Here's how the part is built. I have some questions about the finished solid (model axes, mm). Face numbers are marked on the shaded views. Round coordinates to 2 decimals unless told otherwise and drop trailing zeros. Loops run counter-clockwise (first coordinate to the right, second up) from the corner with the lowest first, then second, coordinate; pieces in that order, holes last. Notation, with made-up numbers: (60, -19) -> (107, -19) arc R13 ccw to (107, -5) -> close; hole circle Ø1 at (-15, 0). An arc over 180 degrees is marked (long way). Use CSV: the item, a comma, the result in double quotes. Start each with the question number.
from build123d import *

# Parameters (mm, degrees)
SKETCH3_R          = 2
CUT_EXTRUDE1_DEPTH = 5


with BuildPart() as part:
    # Sketch1 → Revolve1 (revolve)
    with BuildSketch(Plane.XY):
        Polygon((-26.75, 0), (-26.400045346, 4), (-20, 4), (-20, 0), align=None)
    revolve(axis=Axis((0, 0, 0), (0, 1, 0)))

    # Sketch3 → Cut-Extrude1 (cut, through all)
    with BuildSketch(Plane.XZ):
        with Locations((-16.263455967, 16.263455967)):
            Circle(SKETCH3_R)
        with Locations((16.263455967, 16.263455967)):
            Circle(SKETCH3_R)
        with Locations((-16.263455967, -16.263455967)):
            Circle(SKETCH3_R)
        with Locations((16.263455967, -16.263455967)):
            Circle(SKETCH3_R)
    extrude(amount=-CUT_EXTRUDE1_DEPTH, mode=Mode.SUBTRACT)


solid = part.part
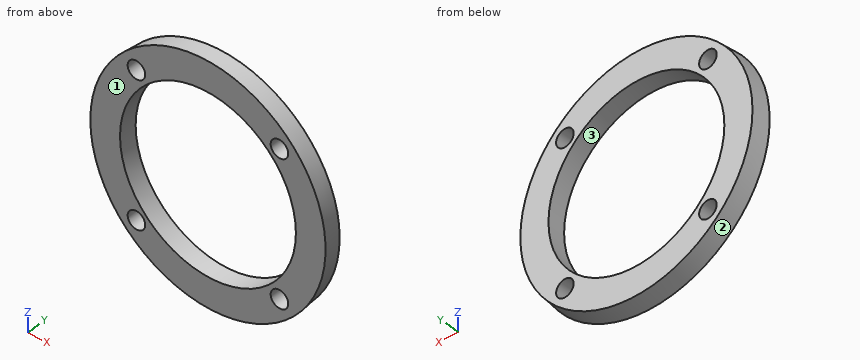
Q1. I need wall thicknesses on line 1 along Z through (x, y) = (-16.5, 0.65); line 2 along X through (y, z) = (0.2, 13.5); line 3 along Z through (x, y) = (9, 3.6). Which ranges of each line are inside material? Lowest first, please.
Q2. I want a section at A-A, the plane x = 0. List the corners of the cut face in (y, z) for me, then the cut area to 3 significant figures.
Q3. I want a section at B-B, the plane z = 0. List the corners of the cut face in (x, y) for me.
Q4. If we mould it in two halves opening along X, with no side actions, what happens to the marked faces 1, 2 and 3? For each: pulls with the +X half, pulls with the -X half, needs draft (parallel to the pull), parting line crosses it, or undercut.
Q5. Will these pins go through, and if not, where does the flat tip stop? pin 1 Ø5 at (x, z) = (15.5, -6.5) entering from +Y; pin 2 Ø2 at (x, y) = (-18.5, 3) entering from -Z; pin 3 Ø1.5 at (x, y) = (12, 3) entering from +Z; pin 4 Ø1.5 at (x, y) = (-8.5, 1.5) entering from -Z.
Q6. I want a section at D-D, the plane z = -17.5. Count the separate pieces of the cut face and the enclosed holes in it, then the cut area to 3 significant figures.
Q7. I want a section at C-C, the plane y = 2.9. List the corners of the cut face in (x, z) for me, then the cut area to 3 significant figures.
Values found:
1,line 1,"-20.98 to -18.25, -14.28 to -11.3, 11.3 to 14.28, 18.25 to 20.98"
1,line 2,"-23.07 to -14.76, 14.76 to 23.07"
1,line 3,"-24.86 to -17.86, 17.86 to 24.86"
2,outline,"(0, -26.75) -> (4, -26.4) -> (4, -20) -> (0, -20) -> close; (0, 20) -> (4, 20) -> (4, 26.4) -> (0, 26.75) -> close"
2,area,"52.6 mm2"
3,outline,"(-26.75, 0) -> (-20, 0) -> (-20, 4) -> (-26.4, 4) -> close; (20, 0) -> (26.75, 0) -> (26.4, 4) -> (20, 4) -> close"
4,face 1,"needs draft"
4,face 2,"parting line crosses it"
4,face 3,"undercut"
5,pin 1,"through"
5,pin 2,"z = -19.89"
5,pin 3,"z = 23.99"
5,pin 4,"z = -25.48"
6,separate pieces,"4"
6,enclosed holes,"0"
6,area,"57.4 mm2"
7,outline,"circle Ø52.99 at (0, 0); hole circle Ø40 at (0, 0); hole circle Ø4 at (-16.26, -16.26); hole circle Ø4 at (-16.26, 16.26); hole circle Ø4 at (16.26, -16.26); hole circle Ø4 at (16.26, 16.26)"
7,area,"899 mm2"
